```python
from build123d import *

# Parameters (mm, degrees)
F0_W     = 215
F0_H     = 68
F1_DEPTH = 12
F2_W     = 3
F2_H     = 5.623123
F3_DEPTH = 300


with BuildPart() as f1:
    # F0 (on Right) → F1 (new body)
    with BuildSketch(Plane.YZ):
        Rectangle(F0_W, F0_H)
    extrude(amount=F1_DEPTH)

    # F2 (on face) → F3 (cut)
    with BuildSketch(Plane(origin=(0, 107.5, 0), x_dir=(-1, 0, 0), z_dir=(0, 1, 0))):
        with Locations((-10.5, 25.16836)):
            Rectangle(F2_W, F2_H)
    extrude(amount=-F3_DEPTH, mode=Mode.SUBTRACT)


solid = f1.part
```
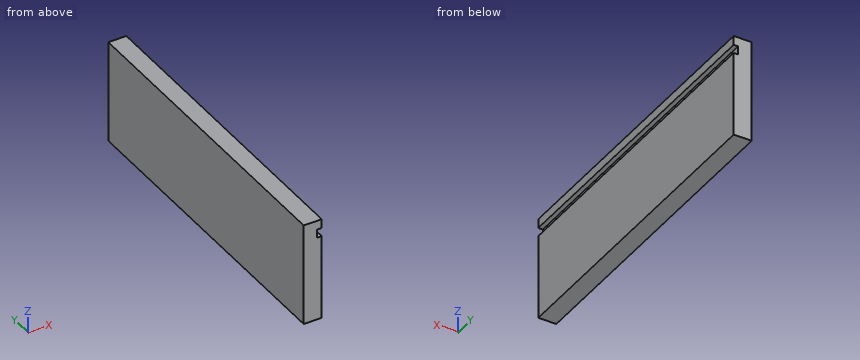
Geometry: final body of the model. Coordinates: model frame, mm. Round coordinates to 2 decimals unless told otherwise and drop trailing zeros. Order: outer loops, then holes, each group sorted by start corner. A loop starts at its lowest first (then second) coordinate and runs counter-clockwise, first axis right, second up. Notation, with made-up numbers: (46.5, 53.5) - (75.5, 53.5) arc R25 cw to (75.5, 90.5) - close; hole circle Ø7 at (-9.5, 89). An arc over 180 degrees is marked (long way). Write item = value, one per line. Start each with the question number.
Q1. Cut plane A-A on y = 12. Return the cut outline in (x, z), and give its area (3 significant figures).
Q2. Pin query (flat end, axial travel): pin 1 (1.7 mm diameter, centred on y = -17, z = 25.5, fed in from +X). Return the tip coordinate at first contact, or that it passes through.
Q3. Ray query, line 1 (Z direction, x = 10.75, y = -5.5); line 2 (X direction, y = -37, z = 23). Return the intervals inside material, ascending. Write a range as from..to.
Outcome:
q1.outline = (0, -34) - (12, -34) - (12, 22.36) - (9, 22.36) - (9, 27.98) - (12, 27.98) - (12, 34) - (0, 34) - close
q1.area = 799 mm^2
q2.pin_1 = 9
q3.line_1 = -34..22.36, 27.98..34
q3.line_2 = 0..9
